Input: part model. Units: mm. Frame: model coordinates. Face numbers are marked on the shaded views. A direction names the side the tool comes from. Give positions to 0.01 mm unless a question says otherwise; leave off trailing zeros. Loops run counter-clockwise (first coordinate to the right, second up) from the corner with the lowest first, then second, coordinate; pieces in that order, holes last. Notation, with made-up numbers: (70, 13.5) - (121, 13.5) arc R18 cw to (121, 37.5) - close; hole circle Ø11 at (-22, -1.5). An arc over 180 degrees is marked (long way). Answer as a JSON object with one key per item and string values.
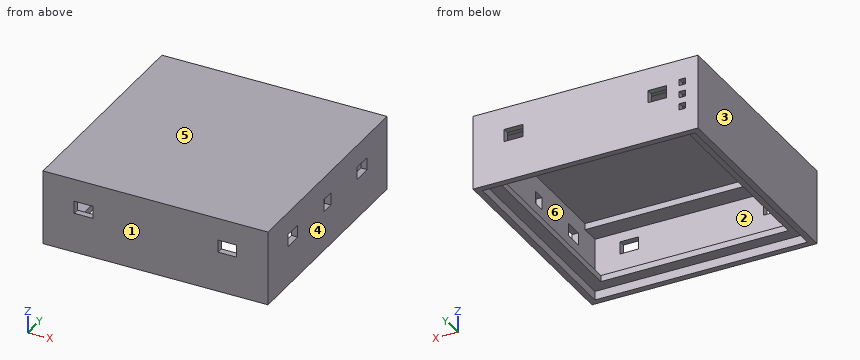
from build123d import *

# Parameters (mm, degrees)
SKETCH1_W            = 180
SKETCH1_H            = 180
BOSS_EXTRUDE1_DEPTH  = 10
SKETCH2_W            = 180
SKETCH2_H            = 180
SKETCH2_W_2          = 160
SKETCH2_H_2          = 160
BOSS_EXTRUDE2_DEPTH  = 80
SKETCH3_W            = 160
SKETCH3_H            = 20
BOSS_EXTRUDE4_DEPTH  = 20
SKETCH5_W            = 20
SKETCH5_H            = 180
CUT_EXTRUDE1_DEPTH   = 300
SKETCH6_W            = 160
SKETCH6_H            = 20
CUT_EXTRUDE2_DEPTH   = 5
SKETCH9_W            = 160
SKETCH9_H            = 15
BOSS_EXTRUDE6_DEPTH  = 10
SKETCH11_W           = 28
SKETCH11_H           = 77
CUT_EXTRUDE4_DEPTH   = 10
SKETCH13_W           = 10
SKETCH13_H           = 10
CUT_EXTRUDE5_DEPTH   = 10
SKETCH15_W           = 10
SKETCH15_H           = 180
BOSS_EXTRUDE7_DEPTH  = 30
SKETCH16_W           = 10
SKETCH16_H           = 15
CUT_EXTRUDE6_DEPTH   = 30
SKETCH17_W           = 10
SKETCH17_H           = 10
CUT_EXTRUDE7_DEPTH   = 300
SKETCH22_W           = 20.069553575
SKETCH22_H           = 29.294084881
BOSS_EXTRUDE8_DEPTH  = 10
SKETCH23_W           = 10
SKETCH23_H           = 10
CUT_EXTRUDE11_DEPTH  = 10
SKETCH24_W           = 180
SKETCH24_H           = 30
CUT_EXTRUDE12_DEPTH  = 300
SKETCH26_W           = 18
SKETCH26_H           = 77
BOSS_EXTRUDE9_DEPTH  = 10
SKETCH27_W           = 160
SKETCH27_H           = 160
CUT_EXTRUDE13_DEPTH  = 10
SKETCH28_W           = 180
SKETCH28_H           = 7.5
BOSS_EXTRUDE10_DEPTH = 180
SKETCH29_W           = 160
SKETCH29_H           = 10
BOSS_EXTRUDE11_DEPTH = 5
SKETCH34_W           = 170
SKETCH34_H           = 170
CUT_EXTRUDE14_DEPTH  = 40
SKETCH35_W           = 180
SKETCH35_H           = 180
SKETCH35_W_2         = 170
SKETCH35_H_2         = 170
BOSS_EXTRUDE13_DEPTH = 20
SKETCH36_W           = 180
SKETCH36_H           = 5
BOSS_EXTRUDE14_DEPTH = 180
SKETCH37_W           = 180
SKETCH37_H           = 180
SKETCH37_W_2         = 170
SKETCH37_H_2         = 170
BOSS_EXTRUDE15_DEPTH = 40
SKETCH38_W           = 170
SKETCH38_H           = 15
BOSS_EXTRUDE16_DEPTH = 5
SKETCH39_W           = 10
SKETCH39_H           = 15
SKETCH39_H_2         = 10
CUT_EXTRUDE15_DEPTH  = 5
SKETCH40_W           = 15
SKETCH40_H           = 10
CUT_EXTRUDE16_DEPTH  = 300
SKETCH44_W           = 170
SKETCH44_H           = 170
SKETCH44_W_2         = 150
SKETCH44_H_2         = 150
BOSS_EXTRUDE17_DEPTH = 5
SKETCH45_W           = 5
SKETCH45_H           = 5
CUT_EXTRUDE17_DEPTH  = 5
SKETCH46_W           = 15
SKETCH46_H           = 10
CUT_EXTRUDE18_DEPTH  = 300


with BuildPart() as part:
    # Sketch1 → Boss-Extrude1 (new body)
    with BuildSketch(Plane.XY):
        with Locations((90, 90)):
            Rectangle(SKETCH1_W, SKETCH1_H)
    extrude(amount=BOSS_EXTRUDE1_DEPTH)

    # Sketch2 → Boss-Extrude2 (add)
    with BuildSketch(Plane.XY.offset(10)):
        with Locations((90, 90)):
            Rectangle(SKETCH2_W, SKETCH2_H)
        with Locations((90, 90)):
            Rectangle(SKETCH2_W_2, SKETCH2_H_2, mode=Mode.SUBTRACT)
    extrude(amount=BOSS_EXTRUDE2_DEPTH)

    # Sketch3 → Boss-Extrude4 (add)
    with BuildSketch(Plane.XY.offset(10)):
        with Locations((90, 20)):
            Rectangle(SKETCH3_W, SKETCH3_H)
        with Locations((90, 160)):
            Rectangle(SKETCH3_W, SKETCH3_H)
    extrude(amount=BOSS_EXTRUDE4_DEPTH)

    # Sketch5 → Cut-Extrude1 (cut)
    with BuildSketch(Plane(origin=(180, 0, 0), x_dir=(0, 0, -1), z_dir=(1, 0, 0))):
        with Locations((-80, 90)):
            Rectangle(SKETCH5_W, SKETCH5_H)
    extrude(amount=-CUT_EXTRUDE1_DEPTH, mode=Mode.SUBTRACT)

    # Sketch6 → Cut-Extrude2 (cut)
    with BuildSketch(Plane.XY.offset(30)):
        with Locations((90, 160)):
            Rectangle(SKETCH6_W, SKETCH6_H)
        with Locations((90, 20)):
            Rectangle(SKETCH6_W, SKETCH6_H)
    extrude(amount=-CUT_EXTRUDE2_DEPTH, mode=Mode.SUBTRACT)

    # Sketch9 → Boss-Extrude6 (add)
    with BuildSketch(Plane.XY.offset(62)):
        with Locations((90, 17.5)):
            Rectangle(SKETCH9_W, SKETCH9_H)
        with Locations((90, 162.5)):
            Rectangle(SKETCH9_W, SKETCH9_H)
    extrude(amount=-BOSS_EXTRUDE6_DEPTH)

    # Sketch11 → Cut-Extrude4 (cut)
    with BuildSketch(Plane.ZY):
        with Locations((34, 83.5)):
            Rectangle(SKETCH11_W, SKETCH11_H)
    extrude(amount=-CUT_EXTRUDE4_DEPTH, mode=Mode.SUBTRACT)

    # Sketch13 → Cut-Extrude5 (cut)
    with BuildSketch(Plane(origin=(180, 0, 0), x_dir=(0, 0, -1), z_dir=(1, 0, 0))):
        with Locations((-45.269958147, 35)):
            Rectangle(SKETCH13_W, SKETCH13_H)
        with Locations((-45.269958147, 145)):
            Rectangle(SKETCH13_W, SKETCH13_H)
        with Locations((-45.269958147, 90)):
            Rectangle(SKETCH13_W, SKETCH13_H)
    extrude(amount=-CUT_EXTRUDE5_DEPTH, mode=Mode.SUBTRACT)

    # Sketch15 → Boss-Extrude7 (add)
    with BuildSketch(Plane.XY.offset(70)):
        with Locations((175, 90)):
            Rectangle(SKETCH15_W, SKETCH15_H)
    extrude(amount=-BOSS_EXTRUDE7_DEPTH)

    # Sketch16 → Cut-Extrude6 (cut)
    with BuildSketch(Plane(origin=(180, 0, 0), x_dir=(0, 0, -1), z_dir=(1, 0, 0))):
        with Locations((-45, 37.5)):
            Rectangle(SKETCH16_W, SKETCH16_H)
        with Locations((-45, 90)):
            Rectangle(SKETCH16_W, SKETCH16_H)
        with Locations((-45, 142.5)):
            Rectangle(SKETCH16_W, SKETCH16_H)
    extrude(amount=-CUT_EXTRUDE6_DEPTH, mode=Mode.SUBTRACT)

    # Sketch17 → Cut-Extrude7 (cut)
    with BuildSketch(Plane(origin=(0, 180, 0), x_dir=(1, 0, 0), z_dir=(0, 1, 0))):
        with Locations((25, -45)):
            Rectangle(SKETCH17_W, SKETCH17_H)
        with Locations((155, -45)):
            Rectangle(SKETCH17_W, SKETCH17_H)
    extrude(amount=-CUT_EXTRUDE7_DEPTH, mode=Mode.SUBTRACT)

    # Sketch22 → Boss-Extrude8 (add)
    with BuildSketch(Plane(origin=(180, 0, 0), x_dir=(0, 0, -1), z_dir=(1, 0, 0))):
        with Locations((-44.930981983, 90.571261677)):
            Rectangle(SKETCH22_W, SKETCH22_H)
    extrude(amount=-BOSS_EXTRUDE8_DEPTH)

    # Sketch23 → Cut-Extrude11 (cut)
    with BuildSketch(Plane.XZ):
        with Locations((25, 25)):
            Rectangle(SKETCH23_W, SKETCH23_H)
    extrude(amount=-CUT_EXTRUDE11_DEPTH, mode=Mode.SUBTRACT)

    # Sketch24 → Cut-Extrude12 (cut)
    with BuildSketch(Plane(origin=(0, 180, 0), x_dir=(1, 0, 0), z_dir=(0, 1, 0))):
        with Locations((90, -15)):
            Rectangle(SKETCH24_W, SKETCH24_H)
    extrude(amount=-CUT_EXTRUDE12_DEPTH, mode=Mode.SUBTRACT)

    # Sketch26 → Boss-Extrude9 (add)
    with BuildSketch(Plane.ZY):
        with Locations((39, 83.5)):
            Rectangle(SKETCH26_W, SKETCH26_H)
    extrude(amount=-BOSS_EXTRUDE9_DEPTH)

    # Sketch27 → Cut-Extrude13 (cut)
    with BuildSketch(Plane.XY.offset(62)):
        with Locations((90, 90)):
            Rectangle(SKETCH27_W, SKETCH27_H)
    extrude(amount=-CUT_EXTRUDE13_DEPTH, mode=Mode.SUBTRACT)

    # Sketch28 → Boss-Extrude10 (add)
    with BuildSketch(Plane(origin=(0, 180, 0), x_dir=(1, 0, 0), z_dir=(0, 1, 0))):
        with Locations((90, -66.25)):
            Rectangle(SKETCH28_W, SKETCH28_H)
    extrude(amount=-BOSS_EXTRUDE10_DEPTH)

    # Sketch29 → Boss-Extrude11 (add)
    with BuildSketch(Plane(origin=(0, 0, 62.5), x_dir=(-1, 0, 0), z_dir=(0, 0, -1))):
        with Locations((-90, 165)):
            Rectangle(SKETCH29_W, SKETCH29_H)
        with Locations((-90, 15)):
            Rectangle(SKETCH29_W, SKETCH29_H)
    extrude(amount=BOSS_EXTRUDE11_DEPTH)

    # Sketch34 → Cut-Extrude14 (cut)
    with BuildSketch(Plane(origin=(0, 0, 30), x_dir=(-1, 0, 0), z_dir=(0, 0, -1))):
        with Locations((-90, 90)):
            Rectangle(SKETCH34_W, SKETCH34_H)
    extrude(amount=-CUT_EXTRUDE14_DEPTH, mode=Mode.SUBTRACT)

    # Sketch35 → Boss-Extrude13 (add)
    with BuildSketch(Plane.XY.offset(70)):
        with Locations((90, 90)):
            Rectangle(SKETCH35_W, SKETCH35_H)
        with Locations((90, 90)):
            Rectangle(SKETCH35_W_2, SKETCH35_H_2, mode=Mode.SUBTRACT)
    extrude(amount=BOSS_EXTRUDE13_DEPTH)

    # Sketch36 → Boss-Extrude14 (add)
    with BuildSketch(Plane.XZ):
        with Locations((90, 87.5)):
            Rectangle(SKETCH36_W, SKETCH36_H)
    extrude(amount=-BOSS_EXTRUDE14_DEPTH)

    # Sketch37 → Boss-Extrude15 (add)
    with BuildSketch(Plane(origin=(0, 0, 30), x_dir=(-1, 0, 0), z_dir=(0, 0, -1))):
        with Locations((-90, 90)):
            Rectangle(SKETCH37_W, SKETCH37_H)
        with Locations((-90, 90)):
            Rectangle(SKETCH37_W_2, SKETCH37_H_2, mode=Mode.SUBTRACT)
    extrude(amount=-BOSS_EXTRUDE15_DEPTH)

    # Sketch38 → Boss-Extrude16 (add)
    with BuildSketch(Plane(origin=(0, 0, 85), x_dir=(-1, 0, 0), z_dir=(0, 0, -1))):
        with Locations((-90, 167.5)):
            Rectangle(SKETCH38_W, SKETCH38_H)
        with Locations((-90, 12.5)):
            Rectangle(SKETCH38_W, SKETCH38_H)
    extrude(amount=BOSS_EXTRUDE16_DEPTH)

    # Sketch39 → Cut-Extrude15 (cut)
    with BuildSketch(Plane(origin=(180, 0, 0), x_dir=(0, 0, -1), z_dir=(1, 0, 0))):
        with Locations((-67, 142.5)):
            Rectangle(SKETCH39_W, SKETCH39_H)
        with Locations((-67, 37.5)):
            Rectangle(SKETCH39_W, SKETCH39_H)
        with Locations((-67, 90)):
            Rectangle(SKETCH39_W, SKETCH39_H_2)
    extrude(amount=-CUT_EXTRUDE15_DEPTH, mode=Mode.SUBTRACT)

    # Sketch40 → Cut-Extrude16 (cut)
    with BuildSketch(Plane(origin=(0, 180, 0), x_dir=(1, 0, 0), z_dir=(0, 1, 0))):
        with Locations((32.5, -67)):
            Rectangle(SKETCH40_W, SKETCH40_H)
    extrude(amount=-CUT_EXTRUDE16_DEPTH, mode=Mode.SUBTRACT)

    # Sketch44 → Boss-Extrude17 (add)
    with BuildSketch(Plane(origin=(0, 0, 37), x_dir=(-1, 0, 0), z_dir=(0, 0, -1))):
        with Locations((-90, 90)):
            Rectangle(SKETCH44_W, SKETCH44_H)
        with Locations((-90, 90)):
            Rectangle(SKETCH44_W_2, SKETCH44_H_2, mode=Mode.SUBTRACT)
    extrude(amount=-BOSS_EXTRUDE17_DEPTH)

    # Sketch45 → Cut-Extrude17 (cut)
    with BuildSketch(Plane(origin=(0, 180, 0), x_dir=(1, 0, 0), z_dir=(0, 1, 0))):
        with Locations((12.5, -61.614476268)):
            Rectangle(SKETCH45_W, SKETCH45_H)
        with Locations((12.5, -51.614476268)):
            Rectangle(SKETCH45_W, SKETCH45_H)
        with Locations((12.5, -71.614476268)):
            Rectangle(SKETCH45_W, SKETCH45_H)
    extrude(amount=-CUT_EXTRUDE17_DEPTH, mode=Mode.SUBTRACT)

    # Sketch46 → Cut-Extrude18 (cut)
    with BuildSketch(Plane(origin=(0, 180, 0), x_dir=(1, 0, 0), z_dir=(0, 1, 0))):
        with Locations((147.5, -67.241667744)):
            Rectangle(SKETCH46_W, SKETCH46_H)
    extrude(amount=-CUT_EXTRUDE18_DEPTH, mode=Mode.SUBTRACT)


solid = part.part
Item 1: Access query for the marked faces 5 and 6. Directions: +Z, -Z, +X, -X, +Y, -Y. A direction counts if a zero-diameter tool reaches every point of the face in a straight line with its end or side. Return the directions, or none.
Geometry check:
{"face 5": "+Z, +X, -X, +Y, -Y", "face 6": "none"}
Item 2: Contact query for a flat-ended pin moving along its axis: P1, Ø8, axis at y = 21, z = 36.5, coming from the -X side. Output: stop coordinate, or through.
Geometry check:
{"P1": "stops at x = 0"}
Item 3: Mould query, pull axis X, two halves, no side actions, for the marked faces 1, 2, 3 and 4. Classes: released by +X, released by -X, zero draft, split by the parting line, or undercut.
Geometry check:
{"face 1": "zero draft", "face 2": "undercut", "face 3": "released by -X", "face 4": "released by +X"}
Item 4: Cut plane A-A (y = 35.5). Return loops of the section in (x, z), then the cut area to 3 significant figures.
Geometry check:
{"outline": "(0, 30) - (5, 30) - (5, 37) - (15, 37) - (15, 42) - (5, 42) - (5, 85) - (175, 85) - (175, 72) - (180, 72) - (180, 90) - (0, 90) - close; (165, 37) - (175, 37) - (175, 30) - (180, 30) - (180, 62) - (175, 62) - (175, 42) - (165, 42) - close", "area": "1,500 mm2"}
Item 5: Cut plane B-B (x = 147). Return loops of the section in (y, z).
Geometry check:
{"outline": "(0, 30) - (5, 30) - (5, 37) - (15, 37) - (15, 42) - (5, 42) - (5, 62.24) - (0, 62.24) - close; (0, 72.24) - (5, 72.24) - (5, 80) - (20, 80) - (20, 85) - (160, 85) - (160, 80) - (175, 80) - (175, 72.24) - (180, 72.24) - (180, 90) - (0, 90) - close; (165, 37) - (175, 37) - (175, 30) - (180, 30) - (180, 62.24) - (175, 62.24) - (175, 42) - (165, 42) - close"}
Item 6: Cut plane D-D (x = 17.5). Return loops of the section in (y, z).
Geometry check:
{"outline": "(0, 30) - (5, 30) - (5, 37) - (15, 37) - (15, 42) - (5, 42) - (5, 80) - (20, 80) - (20, 85) - (160, 85) - (160, 80) - (175, 80) - (175, 42) - (165, 42) - (165, 37) - (175, 37) - (175, 30) - (180, 30) - (180, 90) - (0, 90) - close"}
Item 7: Material intervals for line 1 (X direction, y = 124.5, z = 63); line 2 (Y direction, x = 39, z = 84.5), sorted ascending. Write a range as [from, to].
Geometry check:
{"line 1": "x = [0, 5], [175, 180]", "line 2": "y = [0, 20], [160, 180]"}
Item 8: Cut plane C-C (y = 157). Return loops of the section in (x, z).
Geometry check:
{"outline": "(0, 30) - (5, 30) - (5, 37) - (15, 37) - (15, 42) - (5, 42) - (5, 85) - (175, 85) - (175, 42) - (165, 42) - (165, 37) - (175, 37) - (175, 30) - (180, 30) - (180, 90) - (0, 90) - close"}
